Design review of the part built by this model. Coordinates are the model's own, in mm. Face numbers are marked on the shaded views. Coordinates: 2 decimals unless noted, no trailing zeros. Order: outer loops, then holes, each group sorted by start corner. A loop starts at its lowest first (then second) coordinate and runs counter-clockwise, first axis right, second up. Notation, with made-up numbers: (80.5, 50.25) - (133.5, 50.25) arc R36 ccw to (133.5, 89.25) - close; hole circle Ø4 at (-12.75, 85). An arc over 180 degrees is marked (long way). Write each question's results on one line, items separated by ' | '. Start each with the question number.
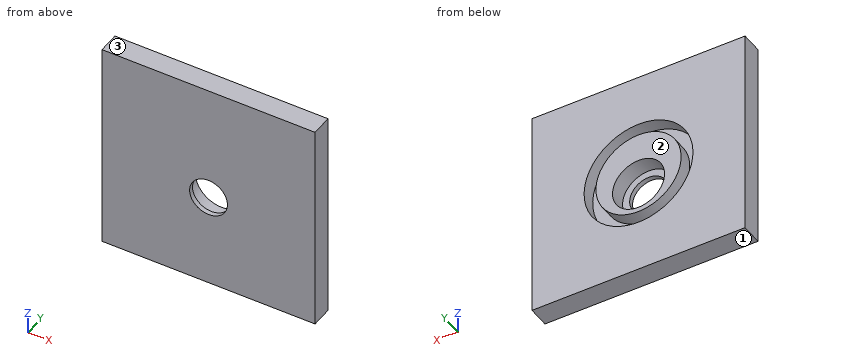
```python
from build123d import *

# Parameters (mm, degrees)
SKETCH_1_W          = 45
SKETCH_1_H          = 45
EXTRUDE_1_DEPTH     = 4.5
SKETCH_2_R          = 5.5
CUT_EXTRUDE_1_DEPTH = 3.5
SKETCH_3_R          = 4
CUT_EXTRUDE_2_DEPTH = 33.011716605
SKETCH_4_R          = 11.5
SKETCH_4_R_2        = 9
CUT_EXTRUDE_3_DEPTH = 3


with BuildPart() as part:
    # 草图1 → 凸台-拉伸1 (new body)
    with BuildSketch(Plane(origin=(0, 0, 0), x_dir=(1, 0, 0), z_dir=(0, 1, 0))):
        Rectangle(SKETCH_1_W, SKETCH_1_H)
    extrude(amount=EXTRUDE_1_DEPTH)

    # 草图2 → 切除-拉伸1 (cut)
    with BuildSketch(Plane(origin=(0, 4.5, 0), x_dir=(1, 0, 0), z_dir=(0, 1, 0))):
        with Locations(Location((0, 2.5, 0), (0, 0, 270))):
            Circle(SKETCH_2_R)
    extrude(amount=-CUT_EXTRUDE_1_DEPTH, mode=Mode.SUBTRACT)

    # 草图3 → 切除-拉伸2 (cut, through all)
    with BuildSketch(Plane(origin=(0, 1, 0), x_dir=(1, 0, 0), z_dir=(0, 1, 0))):
        with Locations(Location((0, 2.5, 0), (0, 0, 270))):
            Circle(SKETCH_3_R)
    extrude(amount=-CUT_EXTRUDE_2_DEPTH, mode=Mode.SUBTRACT)

    # 草图4 → 切除-拉伸3 (cut)
    with BuildSketch(Plane(origin=(0, 4.5, 0), x_dir=(1, 0, 0), z_dir=(0, 1, 0))):
        with Locations(Location((0, 0, 0), (0, 0, 270))):
            Circle(SKETCH_4_R)
        with Locations(Location((0, 0, 0), (0, 0, 270))):
            Circle(SKETCH_4_R_2, mode=Mode.SUBTRACT)
    extrude(amount=-CUT_EXTRUDE_3_DEPTH, mode=Mode.SUBTRACT)


solid = part.part
```
(1) Take a section at C-C (z = -0.5). State the section outline as (x, y) points, plus the area to 3 significant figures.
(2) Take a section at D-D (x = 10.5). State the section outline as (y, z) points.
(3) Clearance check with a flat-ended pin moving along its axis: pin 1 (7 mm diameter, centred on x = -1, z = -2.5, fed in from +Y). State where the tip first meets the part, or that it passes through.
(4) Take a section at B-B (x = 0). State the section outline as (y, z) points.
(5) To check wall thickness, follow line 1 along X through (y, z) = (2.05, 0); line 2 along X through (y, z) = (0.25, 0.5); line 3 along Z through (x, y) = (3, 3.25). State the ranges of each line that lie inside material, in increasing order. Write a range as [from, to].
(6) Mouldability with a two-part tool opening along Z and no side actions: class the marked faces 1, 2 and 3 as +Z half, -Z half, draft (parallel to the pull), parting line (faces both ways), or undercut.
(7) Take a section at A-A (y = 2.65). State the section outline as (x, z) points, plus the area to 3 significant figures.
Worked out:
1) outline: (-22.5, 0) - (-3.46, 0) - (-3.46, 1) - (-5.12, 1) - (-5.12, 4.5) - (-8.99, 4.5) - (-8.99, 1.5) - (-11.49, 1.5) - (-11.49, 4.5) - (-22.5, 4.5) - close; (3.46, 0) - (22.5, 0) - (22.5, 4.5) - (11.49, 4.5) - (11.49, 1.5) - (8.99, 1.5) - (8.99, 4.5) - (5.12, 4.5) - (5.12, 1) - (3.46, 1) - close | area: 145 mm^2
2) outline: (0, -22.5) - (4.5, -22.5) - (4.5, -4.69) - (1.5, -4.69) - (1.5, 4.69) - (4.5, 4.69) - (4.5, 22.5) - (0, 22.5) - close
3) pin 1: y = 1
4) outline: (0, -22.5) - (4.5, -22.5) - (4.5, -11.5) - (1.5, -11.5) - (1.5, -9) - (4.5, -9) - (4.5, -8) - (1, -8) - (1, -6.5) - (0, -6.5) - close; (0, 1.5) - (1, 1.5) - (1, 3) - (4.5, 3) - (4.5, 9) - (1.5, 9) - (1.5, 11.5) - (4.5, 11.5) - (4.5, 22.5) - (0, 22.5) - close
5) line 1: [-22.5, -11.5], [-9, -4.9], [4.9, 9], [11.5, 22.5] | line 2: [-22.5, -2.65], [2.65, 22.5] | line 3: [-22.5, -11.1], [-8.49, -7.11], [2.11, 8.49], [11.1, 22.5]
6) face 1: -Z half | face 2: draft | face 3: +Z half
7) outline: (-22.5, -22.5) - (22.5, -22.5) - (22.5, 22.5) - (-22.5, 22.5) - close; circle Ø18 at (0, 0); hole circle Ø23 at (0, 0); hole circle Ø11 at (0, -2.5) | area: 1,770 mm^2
